Drawing for the job (mm, zero at the part's lowest x, y, z). Coordinates: 2 decimals unless noted, no trailing zeros. Loops run counter-clockwise (first coordinate to the right, second up) from the corner with the lowest first, then second, coordinate; pieces in that order, holes last.
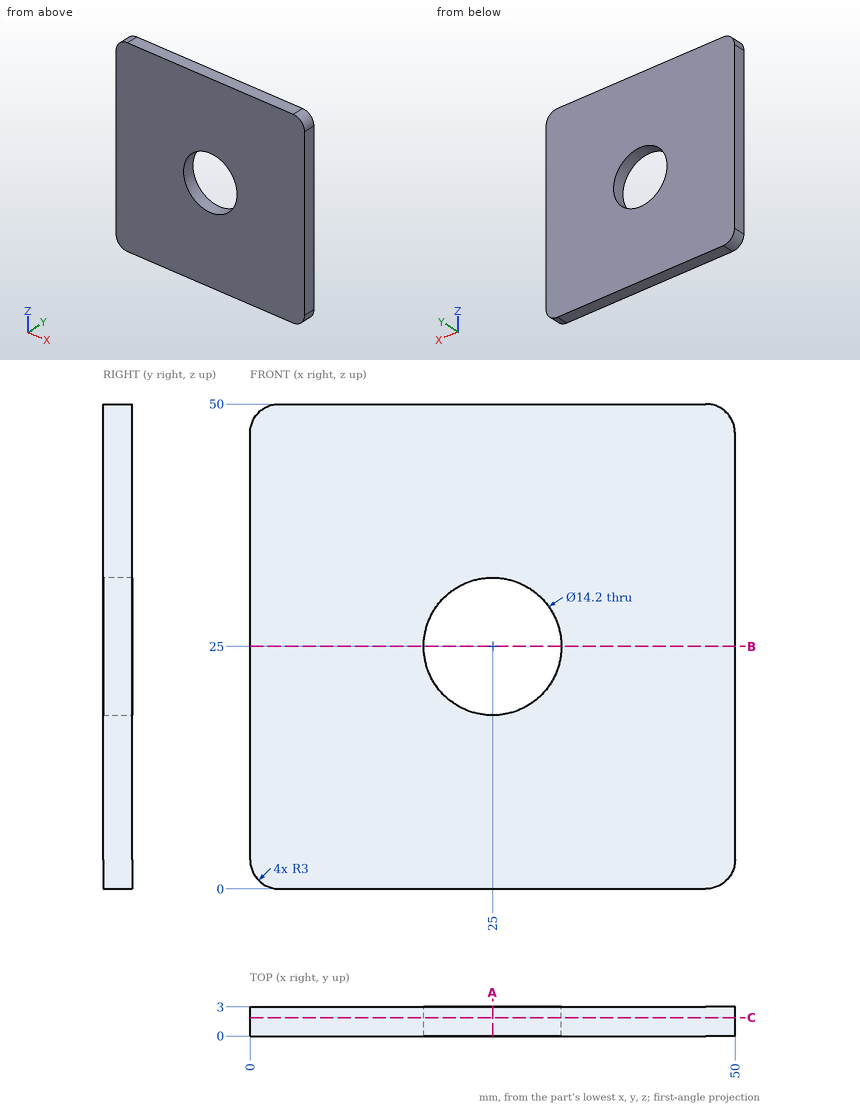
Q1. Probe line 1 (X direction, y = 1.7, z = 25); line 2 (Z direction, x = 27.5, y = 1.8); line 3 (X direction, y = 2.4, z = 20). List the from-to ranges inside material, lowest first.
Q2. Saw through at C-C (y = 1.9). List the corners of the cut face in (x, z).
Q3. Drop a flat-ended pin along its axis: P1, Ø8.5, axis at x = 25, z = 25, coming from the -Y side. Give the stop position or say it passes through.
Q4. Saw through at B-B (z = 25). List the corners of the cut face in (x, y), plus the area to 3 significant figures.
Q5. Saw through at A-A (x = 25). List the corners of the cut face in (y, z), plus the area to 3 significant figures.
Checked values:
1. line 1: x = 0 to 17.9, 32.1 to 50
1. line 2: z = 0 to 18.35, 31.65 to 50
1. line 3: x = 0 to 19.96, 30.04 to 50
2. outline: (0, 3) arc R3 ccw to (3, 0) - (47, 0) arc R3 ccw to (50, 3) - (50, 47) arc R3 ccw to (47, 50) - (3, 50) arc R3 ccw to (0, 47) - close; hole circle Ø14.2 at (25, 25)
3. P1: passes through
4. outline: (0, 0) - (17.9, 0) - (17.9, 3) - (0, 3) - close; (32.1, 0) - (50, 0) - (50, 3) - (32.1, 3) - close
4. area: 107 mm2
5. outline: (0, 0) - (3, 0) - (3, 17.9) - (0, 17.9) - close; (0, 32.1) - (3, 32.1) - (3, 50) - (0, 50) - close
5. area: 107 mm2
